Can you work these out from the model? Positions are in its coordinate system, mm. A direction names the side the tool comes from. Coordinates: 2 decimals unless noted, no trailing zeros. Write each loop counter-clockwise with the first axis right and the second up, starting at its lowest first coordinate (ties: lowest second). Pieces come first, ordered by that corner, then holes.
```python
from build123d import *

# Parameters (mm, degrees)
F0_R     = 57.15
F1_DEPTH = 7.62


with BuildPart() as f1:
    # F0 (on Top) → F1 (new body)
    with BuildSketch(Plane.XY):
        Circle(F0_R)
        with BuildLine():
            ThreePointArc((7.581804, 43.798616), (31.430896, 31.430896), (43.798616, 7.581804))
            ThreePointArc((43.798616, 7.581804), (44.286855, 3.804867), (44.45, 0))
            ThreePointArc((44.45, 0), (44.286855, -3.804867), (43.798616, -7.581804))
            ThreePointArc((43.798616, -7.581804), (31.430896, -31.430896), (7.581804, -43.798616))
            ThreePointArc((7.581804, -43.798616), (0, -44.45), (-7.581804, -43.798616))
            ThreePointArc((-7.581804, -43.798616), (-31.430896, -31.430896), (-43.798616, -7.581804))
            ThreePointArc((-43.798616, -7.581804), (-44.45, 0), (-43.798616, 7.581804))
            ThreePointArc((-43.798616, 7.581804), (-31.430896, 31.430896), (-7.581804, 43.798616))
            ThreePointArc((-7.581804, 43.798616), (0, 44.45), (7.581804, 43.798616))
        make_face(mode=Mode.SUBTRACT)
        with BuildLine():
            ThreePointArc((37.338, -7.581804), (37.909021, -3.81), (38.1, 0))
            ThreePointArc((38.1, 0), (37.909021, 3.81), (37.338, 7.581804))
            ThreePointArc((37.338, 7.581804), (26.940768, 26.940768), (7.581804, 37.338))
            ThreePointArc((7.581804, 37.338), (0, 38.1), (-7.581804, 37.338))
            ThreePointArc((-7.581804, 37.338), (-26.940768, 26.940768), (-37.338, 7.581804))
            ThreePointArc((-37.338, 7.581804), (-38.1, 0), (-37.338, -7.581804))
            ThreePointArc((-37.338, -7.581804), (-26.940768, -26.940768), (-7.581804, -37.338))
            ThreePointArc((-7.581804, -37.338), (0, -38.1), (7.581804, -37.338))
            ThreePointArc((7.581804, -37.338), (26.940768, -26.940768), (37.338, -7.581804))
        make_face()
        with BuildLine():
            ThreePointArc((-7.581804, 37.338), (0, 38.1), (7.581804, 37.338))
            Line((7.581804, 37.338), (7.581804, 43.798616))
            ThreePointArc((7.581804, 43.798616), (0, 44.45), (-7.581804, 43.798616))
            Line((-7.581804, 43.798616), (-7.581804, 37.338))
        make_face()
        with BuildLine():
            ThreePointArc((37.338, 7.581804), (37.909021, 3.81), (38.1, 0))
            ThreePointArc((38.1, 0), (37.909021, -3.81), (37.338, -7.581804))
            Line((37.338, -7.581804), (43.798616, -7.581804))
            ThreePointArc((43.798616, -7.581804), (44.286855, -3.804867), (44.45, 0))
            ThreePointArc((44.45, 0), (44.286855, 3.804867), (43.798616, 7.581804))
            Line((43.798616, 7.581804), (37.338, 7.581804))
        make_face()
        with BuildLine():
            Line((7.581804, -43.798616), (7.581804, -37.338))
            ThreePointArc((7.581804, -37.338), (0, -38.1), (-7.581804, -37.338))
            Line((-7.581804, -37.338), (-7.581804, -43.798616))
            ThreePointArc((-7.581804, -43.798616), (0, -44.45), (7.581804, -43.798616))
        make_face()
        with BuildLine():
            ThreePointArc((-37.338, -7.581804), (-38.1, 0), (-37.338, 7.581804))
            Line((-37.338, 7.581804), (-43.798616, 7.581804))
            ThreePointArc((-43.798616, 7.581804), (-44.45, 0), (-43.798616, -7.581804))
            Line((-43.798616, -7.581804), (-37.338, -7.581804))
        make_face()
    extrude(amount=F1_DEPTH)


solid = f1.part
```
1. We'd pull the mould along Y, two halves only. Please class faces 1 (the face through (26.72, -27.16, 3.76)), 2 (the face through (-1, 1, 7.62)), 3 (the face through (-57.095, 2.513, 3.757)): released by +Y, released by -Y, zero draft, split by the parting line, or undercut.
2. If I drill on L1, parallel to Y at x = -17.5, z = 6.25; L2, parallel to X at y = -8, z = 0.5; L3, parallel to X at y = 9, z = 6.75, over which ranges is the centre line in solid material (lowest first)?
3. If we section it at B-B, the plane x = -20.5: List the corners of the cut face in (y, z) for me.
4. If we section it at A-A, the plane z = 2.75: List the corners of the cut face in (x, y) for me.
5. If we section it at C-C, the plane x = 42: List the corners of the cut face in (y, z) for me, plus the area to 3 significant figures.
6. If we section it at D-D, the plane y = 49: List the corners of the cut face in (x, z) for me.
7. Which directions (+Z, -Z, +X, -X, +Y, -Y) give clear straight access to the entire face, cutting with the end or side of a thin tool? Please do faces 4 (the face through (7.582, 41, 4)), 5 (the face through (-1, 1, 0)).
8. I'm going to push flat-ended pins straight in: P1, Ø1.9, axis at x = -40, z = 4, coming from the -Y side; P2, Ø3, axis at y = 36, z = 2.5, coming from the -X side; P3, Ø3, axis at y = 39.5, z = 2.5, coming from the -X side. Where does each tip first touch, or does it pass through?
Answers:
1. face 1: undercut
1. face 2: zero draft
1. face 3: split by the parting line
2. L1: y = -54.4 to -40.86, -33.84 to 33.84, 40.86 to 54.4
2. L2: x = -56.59 to -43.72, -37.25 to 37.25, 43.72 to 56.59
2. L3: x = -56.44 to -43.53, -37.02 to 37.02, 43.53 to 56.44
3. outline: (-53.35, 0) - (-39.44, 0) - (-39.44, 7.62) - (-53.35, 7.62) - close; (-32.11, 0) - (32.11, 0) - (32.11, 7.62) - (-32.11, 7.62) - close; (39.44, 0) - (53.35, 0) - (53.35, 7.62) - (39.44, 7.62) - close
4. outline: circle Ø114.3 at (0, 0); hole (-43.8, -7.58) arc R44.45 ccw to (-7.58, -43.8) - (-7.58, -37.34) arc R38.1 cw to (-37.34, -7.58) - close; hole (-43.8, 7.58) - (-37.34, 7.58) arc R38.1 cw to (-7.58, 37.34) - (-7.58, 43.8) arc R44.45 ccw to start; hole (7.58, -43.8) arc R44.45 ccw to (43.8, -7.58) - (37.34, -7.58) arc R38.1 cw to (7.58, -37.34) - close; hole (7.58, 37.34) arc R38.1 cw to (37.34, 7.58) - (43.8, 7.58) arc R44.45 ccw to (7.58, 43.8) - close
5. outline: (-38.76, 0) - (-14.55, 0) - (-14.55, 7.62) - (-38.76, 7.62) - close; (-7.58, 0) - (7.58, 0) - (7.58, 7.62) - (-7.58, 7.62) - close; (14.55, 0) - (38.76, 0) - (38.76, 7.62) - (14.55, 7.62) - close
5. area: 484 mm2
6. outline: (-29.41, 0) - (29.41, 0) - (29.41, 7.62) - (-29.41, 7.62) - close
7. face 4: +Z, -Z
7. face 5: -Z, +X, -X, +Y, -Y
8. P1: stops at y = -41.73
8. P2: stops at x = -45.56
8. P3: stops at x = -42.69
